Check sheet for the modelled part. Datum: model origin and axes. Units: mm. A direction names the side the tool comes from. Give positions to 0.01 mm unless a question says otherwise; leave off trailing zeros. Loops run counter-clockwise (first coordinate to the right, second up) from the corner with the lowest first, then second, coordinate; pieces in that order, holes last. Notation, with made-up numbers: M 10,7.5 L 43,7.5 A16 ccw 43,33.5 Z; hole C 89.5,-12 d9. An arc over 180 degrees is marked long. Write each question's results on one line, items separated by ' | '. Start each with the question number.
1. Tool access check on faces 1 (the flat face through (-2.8, 1.7, -10.7)), 2 (the cylindrical face through (6.02, 5.5, -9.86)), 3 (the cylindrical face through (6.02, 0.86, -16.3)), 4 (the flat face through (9.155, -2, 0)). Record the directions out of +Z, -Z, +X, -X, +Y, -Y that give a thin tool (end or side, any length) a straight path to the whole face; none if there is none.
2. Draft check along Y on faces 5 (the cylindrical face through (5.931, 2.719, -13.726)), 6 (the cylindrical face through (-5.93, 5.5, -14.54)), 7 (the cylindrical face through (-28.638, -2.535, 20.987)). Enter one of: pulls with the +Y half, pulls with the -Y half, needs draft (parallel to the pull), parting line crosses it, or undercut.
3. Go/stop test with flat-tipped pins: pin 1 (4.5 mm diameter, centred on x = -26.5, z = -6, fed in from +Y); pin 2 (2 mm diameter, centred on x = -9, z = 11, fed in from +Y); pin 3 (4 mm diameter, centred on y = 3.2, z = 12.2, fed in from +X); pin 4 (1 mm diameter, centred on x = 20.5, z = -3, fed in from +Y). Record where each tip stops, or that it passes through.
4. Sectioned sample at C-C on x = -0.5. Record the cut outline in (y, z), and give its area (3 significant figures).
5. Sectioned sample at B-B on y = -4. Record the cut outline in (x, z) (3 decimals).
6. Sectioned sample at D-D on z = 7. Give the number of separate pieces and of enclosed holes in the cut face, and give its area (3 significant figures).
7. Material ranges on line 1 along Z through (x, y) = (7.75, 3.2); line 2 along X through (y, z) = (-1, 4.5) (3 decimals); line 3 along X through (y, z) = (-2.25, 6.35) (3 decimals), recorded low to high.
8. Sectioned sample at A-A on x = -13. Record the cut outline in (y, z), and give its area (3 significant figures).
```python
from build123d import *

# Parameters (mm, degrees)
SKETCH053_W     = 59.2
SKETCH053_H     = 43.8
SKETCH053_R     = 1.6
PAD029_DEPTH    = 5
SKETCH054_R     = 3.875
SKETCH054_R_2   = 1.6
PAD030_DEPTH    = 2
SKETCH055_W     = 6.35
SKETCH055_H     = 6.4
PAD031_DEPTH    = 6.4
SKETCH056_W     = 10.79
SKETCH056_H     = 33.8
POCKET025_DEPTH = 5
SKETCH057_R     = 1.6
POCKET026_DEPTH = 19.05
FILLET024_R     = 1.9
FILLET025_R     = 3
FILLET026_R     = 3.2


with BuildPart() as part:
    # Sketch053 → Pad029 (new body)
    with BuildSketch(Plane.XZ):
        Rectangle(SKETCH053_W, SKETCH053_H)
        with Locations((25.725, 6.35)):
            Circle(SKETCH053_R, mode=Mode.SUBTRACT)
        with Locations((-25.725, 6.35)):
            Circle(SKETCH053_R, mode=Mode.SUBTRACT)
        with Locations((-25.725, -6.35)):
            Circle(SKETCH053_R, mode=Mode.SUBTRACT)
        with Locations((25.725, -6.35)):
            Circle(SKETCH053_R, mode=Mode.SUBTRACT)
    extrude(amount=PAD029_DEPTH)

    # Sketch054 (on Face9 of Pad029) → Pad030 (join)
    with BuildSketch(Plane(origin=(0, 0, 0), x_dir=(1, 0, 0), z_dir=(0, 1, 0))):
        with Locations((-25.725, 6.35)):
            Circle(SKETCH054_R)
        with Locations((-25.725, 6.35)):
            Circle(SKETCH054_R_2, mode=Mode.SUBTRACT)
        with Locations((-25.725, -6.35)):
            Circle(SKETCH054_R)
        with Locations((-25.725, -6.35)):
            Circle(SKETCH054_R_2, mode=Mode.SUBTRACT)
        with Locations((25.725, -6.35)):
            Circle(SKETCH054_R)
        with Locations((25.725, -6.35)):
            Circle(SKETCH054_R_2, mode=Mode.SUBTRACT)
        with Locations((25.725, 6.35)):
            Circle(SKETCH054_R)
        with Locations((25.725, 6.35)):
            Circle(SKETCH054_R_2, mode=Mode.SUBTRACT)
    extrude(amount=PAD030_DEPTH)

    # Sketch055 (on Face4 of Pad030) → Pad031 (join)
    with BuildSketch(Plane(origin=(0, 0, 0), x_dir=(1, 0, 0), z_dir=(0, 1, 0))):
        with Locations((5.975, 12.2)):
            Rectangle(SKETCH055_W, SKETCH055_H)
        with Locations((5.975, -12.2)):
            Rectangle(SKETCH055_W, SKETCH055_H)
        with Locations((-5.975, -12.2)):
            Rectangle(SKETCH055_W, SKETCH055_H)
        with Locations((-5.975, 12.2)):
            Rectangle(SKETCH055_W, SKETCH055_H)
    extrude(amount=PAD031_DEPTH)

    # Sketch056 (on Face4 of Pad031) → Pocket025 (cut)
    with BuildSketch(Plane(origin=(0, 0, 0), x_dir=(1, 0, 0), z_dir=(0, 1, 0))):
        with Locations((-14.55, 0)):
            Rectangle(SKETCH056_W, SKETCH056_H)
        with Locations((14.55, 0)):
            Rectangle(SKETCH056_W, SKETCH056_H)
    extrude(amount=-POCKET025_DEPTH, mode=Mode.SUBTRACT)

    # Sketch057 (on Face8 of Pocket025) → Pocket026 (cut)
    with BuildSketch(Plane(origin=(-9.15, 0, 0), x_dir=(0, 0, -1), z_dir=(-1, 0, 0))):
        with Locations((-12.2, -3.2)):
            Circle(SKETCH057_R)
        with Locations((12.2, -3.2)):
            Circle(SKETCH057_R)
    extrude(amount=-POCKET026_DEPTH, mode=Mode.SUBTRACT)

    # Fillet024
    fillet024_edges = [part.edges().sort_by_distance(p)[0] for p in [
        (21.85, 2, 6.35),
        (21.85, 2, -6.35),
        (-29.6, 2, -6.35),
        (-29.6, 2, 6.35),
    ]]
    fillet(fillet024_edges, radius=FILLET024_R)

    # Fillet025
    fillet025_edges = [part.edges().sort_by_distance(p)[0] for p in [
        (5.975, 6.4, -15.4),
        (-5.975, 6.4, -15.4),
        (5.975, 6.4, 9),
        (-5.975, 6.4, 9),
        (5.975, 6.4, 15.4),
        (-5.975, 6.4, 15.4),
        (-5.975, 6.4, -9),
        (5.975, 6.4, -9),
        (5.975, 0, 15.4),
        (-5.975, 0, 15.4),
        (-5.975, 0, -9),
        (5.975, 0, -9),
        (5.975, 0, -15.4),
        (-5.975, 0, -15.4),
        (-5.975, 0, 9),
        (5.975, 0, 9),
    ]]
    fillet(fillet025_edges, radius=FILLET025_R)

    # Fillet026
    fillet026_edges = [part.edges().sort_by_distance(p)[0] for p in [
        (29.6, -2.5, 21.9),
        (29.6, -2.5, -21.9),
        (-29.6, -2.5, -21.9),
        (-29.6, -2.5, 21.9),
    ]]
    fillet(fillet026_edges, radius=FILLET026_R)


solid = part.part
```
Output values:
1) face 1: +Z, -Z, +Y | face 2: +X, -X, +Y | face 3: -Z, +X, -X, +Y | face 4: +Y, -Y
2) face 5: undercut | face 6: pulls with the +Y half | face 7: needs draft
3) pin 1: y = 2 | pin 2: y = 6.4 | pin 3: x = 9.15 | pin 4: y = 0
4) outline: M -5,-21.9 L 0,-21.9 L 0,21.9 L -5,21.9 Z | area: 219 mm2
5) outline: M -29.6,-18.7 A3.2 ccw -26.4,-21.9 L 26.4,-21.9 A3.2 ccw 29.6,-18.7 L 29.6,18.7 A3.2 ccw 26.4,21.9 L -26.4,21.9 A3.2 ccw -29.6,18.7 Z; hole C -25.725,-6.35 d3.2; hole C -25.725,6.35 d3.2; hole M -19.945,-16.9 L -9.155,-16.9 L -9.155,16.9 L -19.945,16.9 Z; hole M 9.155,-16.9 L 19.945,-16.9 L 19.945,16.9 L 9.155,16.9 Z; hole C 25.725,-6.35 d3.2; hole C 25.725,6.35 d3.2
6) separate pieces: 5 | enclosed holes: 0 | area: 177 mm2
7) line 1: -15.4 to -13.8, -10.6 to -9, 9 to 10.6, 13.8 to 15.4 | line 2: -29.6 to -19.945, -9.155 to 9.155, 19.945 to 29.6 | line 3: -29.6 to -27.325, -24.125 to -19.945, -9.155 to 9.155, 19.945 to 24.125, 27.325 to 29.6
8) outline: M -5,-21.9 L 0,-21.9 L 0,-16.9 L -5,-16.9 Z; M -5,16.9 L 0,16.9 L 0,21.9 L -5,21.9 Z | area: 50.0 mm2
